from build123d import *

# Parameters (mm, degrees)
SKETCH2_W            = 22.85
SKETCH2_H            = 22.85
BOSS_EXTRUDE1_DEPTH  = 2
SKETCH3_W            = 4
SKETCH3_H            = 4
BOSS_EXTRUDE2_DEPTH  = 2
M2_CLEARANCE_HOLE1_D = 2.4
CUT_EXTRUDE3_REACH   = 21.299
CUT_EXTRUDE4_REACH   = 21.299
SKETCH8_W            = 4
SKETCH8_H            = 3.2
SKETCH10_W           = 4.95
SKETCH10_H           = 2
SKETCH10_W_2         = 2.01114152
BOSS_EXTRUDE3_DEPTH  = 1.5
SKETCH11_W           = 1
SKETCH11_H           = 4.95
SKETCH11_H_2         = 2.01114152
BOSS_EXTRUDE4_DEPTH  = 4
SKETCH12_W           = 2.993624713
SKETCH12_H           = 2
SKETCH12_W_2         = 12.756375287
BOSS_EXTRUDE5_DEPTH  = 2
SKETCH13_W           = 1
SKETCH13_H           = 2
BOSS_EXTRUDE6_DEPTH  = 7.1
SKETCH15_R           = 1
BOSS_EXTRUDE7_DEPTH  = 2.5
CHAMFER1_SIZE        = 0.5


with BuildPart() as part:
    # Sketch2 → Boss-Extrude1 (new body)
    with BuildSketch(Plane(origin=(0, 0, 0), x_dir=(0, 1, 0), z_dir=(0, 0, 1))):
        Rectangle(SKETCH2_W, SKETCH2_H)
    extrude(amount=BOSS_EXTRUDE1_DEPTH)

    # Sketch3 → Boss-Extrude2 (add)
    with BuildSketch(Plane.XY.offset(2)):
        with Locations((0, 13.425)):
            Rectangle(SKETCH3_W, SKETCH3_H)
        with Locations((0, -13.425)):
            Rectangle(SKETCH3_W, SKETCH3_H)
    extrude(amount=-BOSS_EXTRUDE2_DEPTH)

    # M2 Clearance Hole1 (through all)
    with Locations(Plane.XY.offset(2)):
        with Locations((0, 13.425), (0, -13.425)):
            Hole(M2_CLEARANCE_HOLE1_D / 2)

    # Sketch7 → Cut-Extrude3 (cut, up to next)
    with BuildSketch(Plane.XY.offset(2), mode=Mode.PRIVATE) as cut_extrude3_sk1:
        Polygon((11.425, 8.431375287), (11.425, 1.331375287), (3.325, 1.331375287), (3.325, 1.131375287), (-0.675, 1.131375287), (-0.675, 10.131375287), (3.325, 10.131375287), (3.325, 9.931375287), (8.325, 9.931375287), (8.325, 8.431375287), align=None)
    cut_extrude3_tool1 = extrude(cut_extrude3_sk1.sketch, amount=-CUT_EXTRUDE3_REACH, mode=Mode.PRIVATE) & part.part
    add(cut_extrude3_tool1.solids().sort_by_distance((5.10369, 5.467951, 2))[0], mode=Mode.SUBTRACT)

    # Sketch8 → Cut-Extrude4 (cut, up to next)
    with BuildSketch(Plane.XY.offset(2), mode=Mode.PRIVATE) as cut_extrude4_sk1:
        with Locations((-9.425, -4.875)):
            Rectangle(SKETCH8_W, SKETCH8_H)
    cut_extrude4_tool1 = extrude(cut_extrude4_sk1.sketch, amount=-CUT_EXTRUDE4_REACH, mode=Mode.PRIVATE) & part.part
    add(cut_extrude4_tool1.solids().sort_by_distance((-9.425, -4.875, 2))[0], mode=Mode.SUBTRACT)

    # Sketch10 → Boss-Extrude3 (add)
    with BuildSketch(Plane(origin=(-11.425, 0, 0), x_dir=(0, -1, 0), z_dir=(-1, 0, 0))):
        with Locations((8.95, 1)):
            Rectangle(SKETCH10_W, SKETCH10_H)
        with Locations((2.26942924, 1)):
            Rectangle(SKETCH10_W_2, SKETCH10_H)
    extrude(amount=BOSS_EXTRUDE3_DEPTH)

    # Sketch11 → Boss-Extrude4 (add)
    with BuildSketch(Plane(origin=(0, 0, 0), x_dir=(1, 0, 0), z_dir=(0, 0, -1))):
        with Locations((-12.425, 8.95)):
            Rectangle(SKETCH11_W, SKETCH11_H)
        with Locations((-12.425, 2.26942924)):
            Rectangle(SKETCH11_W, SKETCH11_H_2)
    extrude(amount=BOSS_EXTRUDE4_DEPTH)

    # Sketch12 → Boss-Extrude5 (add)
    with BuildSketch(Plane.YZ.offset(11.425)):
        with Locations((9.928187643, 1)):
            Rectangle(SKETCH12_W, SKETCH12_H)
        with Locations((-5.046812357, 1)):
            Rectangle(SKETCH12_W_2, SKETCH12_H)
    extrude(amount=BOSS_EXTRUDE5_DEPTH)

    # Sketch13 → Boss-Extrude6 (add)
    with BuildSketch(Plane(origin=(0, 1.331375287, 0), x_dir=(-1, 0, 0), z_dir=(0, 1, 0))):
        with Locations((-12.925, 1)):
            Rectangle(SKETCH13_W, SKETCH13_H)
    extrude(amount=BOSS_EXTRUDE6_DEPTH)

    # Sketch15 → Boss-Extrude7 (add)
    with BuildSketch(Plane(origin=(0, 0, 0), x_dir=(1, 0, 0), z_dir=(0, 0, -1))):
        with Locations((-1.425, 4.875)):
            Circle(SKETCH15_R)
        with Locations((6.575, 4.875)):
            Circle(SKETCH15_R)
        with Locations((-7.425, -2.625)):
            Circle(SKETCH15_R)
    extrude(amount=BOSS_EXTRUDE7_DEPTH)

    # Chamfer1
    chamfer1_edges = [part.edges().sort_by_distance(p)[0] for p in [
        (-8.425, 2.625, -2.5),
        (5.575, -4.875, -2.5),
        (-2.425, -4.875, -2.5),
    ]]
    chamfer(chamfer1_edges, length=CHAMFER1_SIZE)


solid = part.part
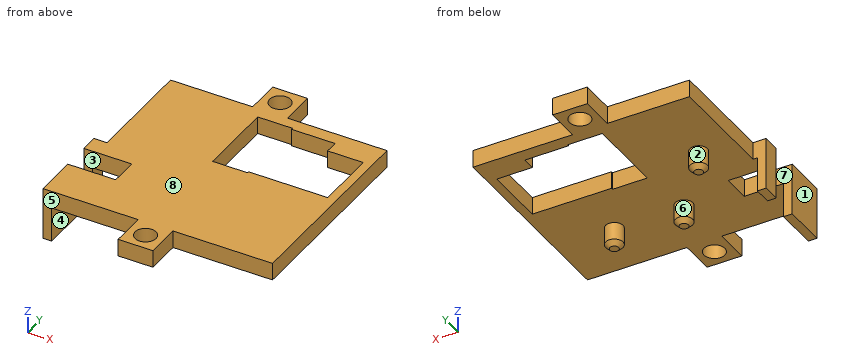
Could you check a few things on this model? Use its own coordinates, in mm. Face numbers are marked on the shaded views. A direction names the side the tool comes from. Round coordinates to 2 decimals unless told otherwise and drop trailing zeros. Write each loop counter-clockwise with the first axis right and the second up, starting at its lowest first coordinate (ties: lowest second). Pieces come first, ordered by that corner, then holes. Notation, with made-up numbers: (-28, 31.5) - (-12, 31.5) arc R18 ccw to (-12, 61.5) - close; hole circle Ø5 at (74.5, 19). An arc over 180 degrees is marked (long way). Use a Markdown table: item, result.
Q1. I want a section at C-C (x = 0). List the corners of the cut face in (y, z) for me (3 decimals).
Output values:
| item | result |
|---|---|
| outline | (-15.425, 0) - (-14.625, 0) - (-14.625, 2) - (-15.425, 2) - close; (-12.225, 0) - (1.131, 0) - (1.131, 2) - (-12.225, 2) - close; (10.131, 0) - (12.225, 0) - (12.225, 2) - (10.131, 2) - close; (14.625, 0) - (15.425, 0) - (15.425, 2) - (14.625, 2) - close |
Q2. For the marked faces 4, 5, 6, 7 and 8, which set-ups out of +Z, -Z, +X, -X, +Y, -Y let a thin tool reach every point of the face, with its end or its side?
Output values:
| item | result |
|---|---|
| face 4 | -Z, +X, +Y, -Y |
| face 5 | +Z, -Z, -X, -Y |
| face 6 | -Z |
| face 7 | +Z, -Z, -X |
| face 8 | +Z, +X, -X, +Y, -Y |
Q3. I want a section at A-A (x = 3.75). List the corners of the cut face in (y, z) for me (3 decimals), plus the area to 3 significant figures.
Output values:
| item | result |
|---|---|
| outline | (-11.425, 0) - (1.331, 0) - (1.331, 2) - (-11.425, 2) - close; (9.931, 0) - (11.425, 0) - (11.425, 2) - (9.931, 2) - close |
| area | 28.5 mm2 |
Q4. For pin 1 (1.6 mm diameter, centred on y = 2, z = 1, fed in from -X) (3 decimals); pin 2 (1 mm diameter, centred on y = 0.5, z = -3, fed in from -X); pin 3 (0.8 mm diameter, centred on x = -12, z = -2.5, fed in from +Y); pin 4 (1.6 mm diameter, centred on y = -13, z = 1, fed in from -X), each with a flat end and sliding along its axis, tell me the tip position at first contact or that it passes through.
Output values:
| item | result |
|---|---|
| pin 1 | x = -11.425 |
| pin 2 | through |
| pin 3 | y = -1.26 |
| pin 4 | x = -2 |
Q5. I want a section at D-D (z = -0.5). List the corners of the cut face in (x, y) for me (3 decimals).
Output values:
| item | result |
|---|---|
| outline | (-12.925, -11.425) - (-11.925, -11.425) - (-11.925, -6.475) - (-12.925, -6.475) - close; (-12.925, -3.275) - (-11.925, -3.275) - (-11.925, -1.264) - (-12.925, -1.264) - close; circle Ø2 at (-7.425, 2.625); circle Ø2 at (-1.425, -4.875); circle Ø2 at (6.575, -4.875) |
Q6. I want a section at B-B (y = 6). List the corners of the cut face in (x, z) for me (3 decimals).
Output values:
| item | result |
|---|---|
| outline | (-11.425, 0) - (-0.675, 0) - (-0.675, 2) - (-11.425, 2) - close; (12.425, 0) - (13.425, 0) - (13.425, 2) - (12.425, 2) - close |
Q7. Please list where these lines run through material, in increasing order: L1, parallel to Y at x = 0, z = 1.6 (3 decimals); L2, parallel to Y at x = -0.5, z = 1.4 (3 decimals); L3, parallel to X at y = 7, z = 0.5 (3 decimals).
Output values:
| item | result |
|---|---|
| L1 | -15.425 to -14.625, -12.225 to 1.131, 10.131 to 12.225, 14.625 to 15.425 |
| L2 | -15.425 to -14.516, -12.334 to 1.131, 10.131 to 12.334, 14.516 to 15.425 |
| L3 | -11.425 to -0.675, 12.425 to 13.425 |
Q8. Thinking about a two-plate mould opening in Y: for the marked faces 1, 2 and 3, which applies, released by +Y, released by -Y, zero draft, split by the parting line, or undercut?
Output values:
| item | result |
|---|---|
| face 1 | zero draft |
| face 2 | split by the parting line |
| face 3 | undercut |
